```python
from build123d import *

# Parameters (mm, degrees)
RESSALTO_EXTRUS_O2_DEPTH = 10
ESBO_O5_R                = 2
CORTE_EXTRUS_O3_DEPTH    = 15
ESBO_O6_W                = 5
ESBO_O6_H                = 16
CORTE_EXTRUS_O4_DEPTH    = 15


with BuildPart() as part:
    # Esboço4 → Ressalto-extrusão2 (new body)
    with BuildSketch(Plane.XY):
        Polygon((-7.5, 20), (-7.5, 4), (-20, 4), (-20, 0), (20, 0), (20, 4), (7.5, 4), (7.5, 20), align=None)
        with BuildLine():
            Line((3.5, 14), (3.5, 10.5))
            ThreePointArc((3.5, 10.5), (0, 7), (-3.5, 10.5))
            Line((-3.5, 10.5), (-3.5, 14))
            ThreePointArc((-3.5, 14), (0, 17.5), (3.5, 14))
        make_face(mode=Mode.SUBTRACT)
    extrude(amount=RESSALTO_EXTRUS_O2_DEPTH)

    # Esboço5 → Corte-extrusão3 (cut)
    with BuildSketch(Plane(origin=(0, 4, 0), x_dir=(1, 0, 0), z_dir=(0, 1, 0))):
        with Locations((-13.75, -5)):
            Circle(ESBO_O5_R)
        with Locations((13.75, -5)):
            Circle(ESBO_O5_R)
    extrude(amount=-CORTE_EXTRUS_O3_DEPTH, mode=Mode.SUBTRACT)

    # Esboço6 → Corte-extrusão4 (cut)
    with BuildSketch(Plane.ZY.offset(7.5)):
        with Locations((7.5, 12)):
            Rectangle(ESBO_O6_W, ESBO_O6_H)
    extrude(amount=-CORTE_EXTRUS_O4_DEPTH, mode=Mode.SUBTRACT)


solid = part.part
```
For this review, take the finished solid that the model builds, in its own axes (mm). A direction names the side the tool comes from. Round coordinates to 2 decimals unless told otherwise and drop trailing zeros. Write each loop counter-clockwise with the first axis right and the second up, starting at its lowest first coordinate (ties: lowest second). Pieces come first, ordered by that corner, then holes. Notation, with made-up numbers: (45, -15) - (71, -15) arc R25 cw to (71, 5) - close; hole circle Ø10 at (63.25, 24). An arc over 180 degrees is marked (long way). Write each question's results on one line, items separated by ' | '.
Item 1: For pin 1 (4 mm diameter, centred on x = -14.5, z = 3.5, fed in from +Y); pin 2 (5 mm diameter, centred on x = -8, z = 4.5, fed in from +Y); pin 3 (1.8 mm diameter, centred on y = 12, z = 3.5, fed in from -X); pin 4 (2.5 mm diameter, centred on y = 12, z = 3, fed in from +X), all flat-tipped, find the tip position at first contact; note any pin that passes through.
Calculated:
pin 1: stops at y = 4 | pin 2: stops at y = 20 | pin 3: stops at x = -7.5 | pin 4: stops at x = 7.5
Item 2: Draft analysis for pull direction X (two halves, no side actions). For faces 4 (the face through (20, 2, 5)), 5 (the face through (0, 7, 2)), 6 (the face through (0, 0, 5)), state which applies: pulls with the +X half, pulls with the -X half, needs draft (parallel to the pull), parting line crosses it, or undercut.
Calculated:
face 4: pulls with the +X half | face 5: undercut | face 6: needs draft
Item 3: For faces 1 (the face through (-3, 8, 5)), 2 (the face through (7.5, 12, 2)), 3 (the face through (-0.1, 17.5, 2.5)), list the 3-axis set-ups (+Z, -Z, +X, -X, +Y, -Y) from which the entire face can be reached by the end or side of a thin tool; tool diameter is ignored.
Calculated:
face 1: +Z, +X, -X, +Y | face 2: +Z, -Z, +X, +Y | face 3: +Z, -Z
Item 4: Take a section at A-A on z = 1. State the section outline as (x, y) points, then the cut area to 3 significant figures.
Calculated:
outline: (-20, 0) - (20, 0) - (20, 4) - (7.5, 4) - (7.5, 20) - (-7.5, 20) - (-7.5, 4) - (-20, 4) - close; hole (-3.5, 10.5) arc R3.5 ccw to (3.5, 10.5) - (3.5, 14) arc R3.5 ccw to (-3.5, 14) - close | area: 337 mm^2
Item 5: Take a section at B-B on x = 13.75. State the section outline as (y, z) points.
Calculated:
outline: (0, 0) - (4, 0) - (4, 3) - (0, 3) - close; (0, 7) - (4, 7) - (4, 10) - (0, 10) - close
Item 6: Take a section at C-C on z = 4. State the section outline as (x, y) points.
Calculated:
outline: (-20, 0) - (-15.48, 0) - (-15.48, 4) - (-20, 4) - close; (-12.02, 0) - (12.02, 0) - (12.02, 4) - (7.5, 4) - (7.5, 20) - (-7.5, 20) - (-7.5, 4) - (-12.02, 4) - close; (15.48, 0) - (20, 0) - (20, 4) - (15.48, 4) - close; hole (-3.5, 10.5) arc R3.5 ccw to (3.5, 10.5) - (3.5, 14) arc R3.5 ccw to (-3.5, 14) - close
Item 7: Take a section at D-D on x = 5.5. State the section outline as (y, z) points.
Calculated:
outline: (0, 0) - (20, 0) - (20, 5) - (4, 5) - (4, 10) - (0, 10) - close
Item 8: To check wall thickness, follow line 1 along X through (y, z) = (1.95, 5); line 2 along Z through (x, y) = (-13.75, 3.1); line 3 along Z through (x, y) = (-5, 12). State the ranges of each line that lie inside material, in increasing order. Write a range as from..to.
Calculated:
line 1: x = -20..-15.75, -11.75..11.75, 15.75..20 | line 2: z = 0..3, 7..10 | line 3: z = 0..5
